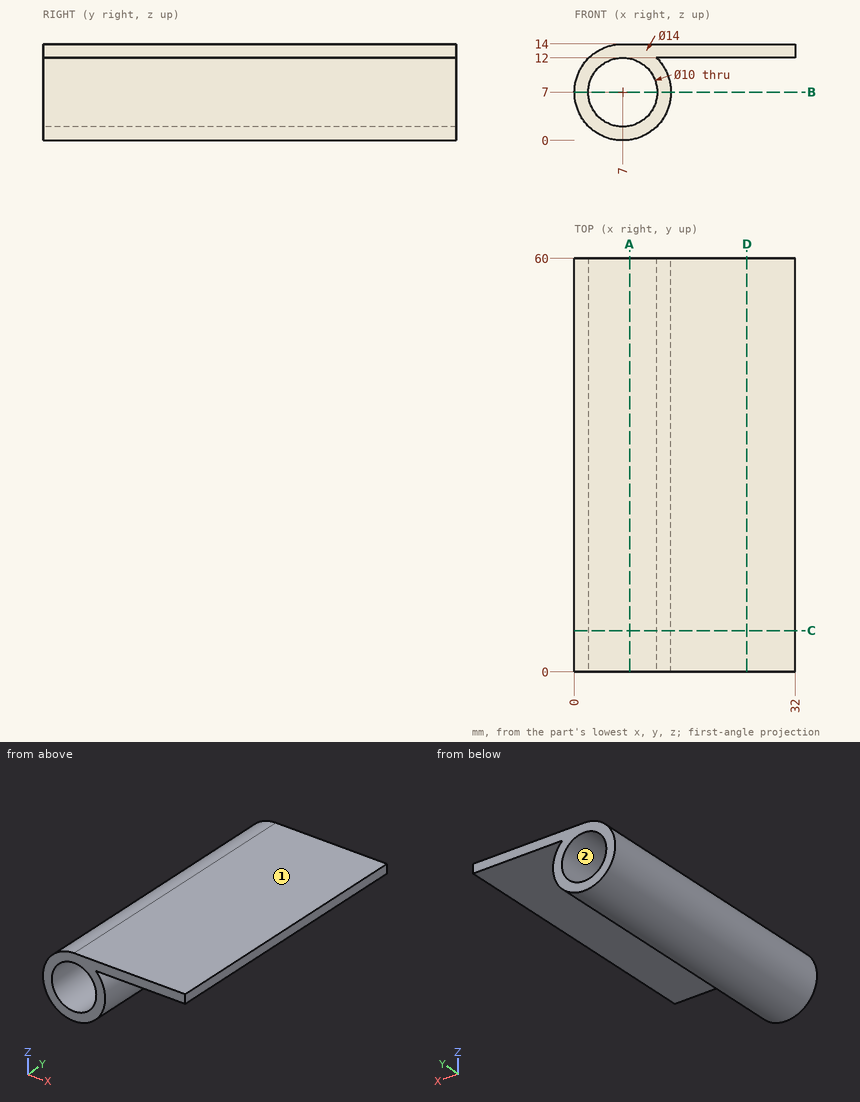
Drawing for the job (mm, zero at the part's lowest x, y, z). Round coordinates to 2 decimals unless told otherwise and drop trailing zeros. Loops run counter-clockwise (first coordinate to the right, second up) from the corner with the lowest first, then second, coordinate; pieces in that order, holes last.
1. Band-saw the part on A-A, the plane x = 8. List the corners of the cut face in (y, z), and give its area (3 significant figures).
Check values:
outline: (0, 0.07) - (60, 0.07) - (60, 2.1) - (0, 2.1) - close; (0, 11.9) - (60, 11.9) - (60, 14) - (0, 14) - close
area: 248 mm2
2. Drop flat-ended pins along their axis: P1, Ø1, axis at x = 8.5, y = 21, coming from the -Z side; P2, Ø5, axis at x = 8.5, y = 16, coming from the -Z side; P3, Ø5, axis at x = 24.5, y = 8, coming from the -Z side; P4, Ø5, axis at y = 23, z = 6.5, coming from the +X side. Give the stop position or say it passes through.
Check values:
P1: stops at z = 0.07
P2: stops at z = 0
P3: stops at z = 12
P4: stops at x = 14
3. Band-saw the part on C-C, the plane y = 6. List the corners of the cut face in (x, z).
Check values:
outline: (7, 14) arc R7 ccw (long way) to (11.9, 12) - (32, 12) - (32, 14) - close; hole circle Ø10 at (7, 7)
4. Band-saw the part on D-D, the plane x = 25. List the corners of the cut face in (y, z).
Check values:
outline: (0, 12) - (60, 12) - (60, 14) - (0, 14) - close
5. Band-saw the part on B-B, the plane z = 7. List the corners of the cut face in (x, y), and give its area (3 significant figures).
Check values:
outline: (0, 0) - (2, 0) - (2, 60) - (0, 60) - close; (12, 0) - (14, 0) - (14, 60) - (12, 60) - close
area: 240 mm2
6. Mould opens along Z. For the marked faces 1 and 2 say: +Z half, -Z half, draft (parallel to the pull), parting line (faces both ways), or undercut.
Check values:
face 1: +Z half
face 2: undercut
7. Wall check: probe 1 along X at (y, z) = (39.5, 7); probe 2 along Z at (x, y) = (28, 5.5). Give the ranges that are in metal, low to high.
Check values:
probe 1: x = 0 to 2, 12 to 14
probe 2: z = 12 to 14
